The listing builds one solid part. Answer for the finished solid, in the listing's coordinates (mm). A direction names the side the tool comes from. Coordinates: 2 decimals unless noted, no trailing zeros. Order: outer loops, then holes, each group sorted by start corner. A loop starts at its lowest first (then second) coordinate and runs counter-clockwise, first axis right, second up. Notation, with made-up numbers: (27.25, 84) -> (79.25, 84) arc R18 ccw to (79.25, 98) -> close; hole circle Ø6 at (24.5, 25). An arc over 180 degrees is marked (long way). Answer in a Markdown table with one row per item. Add a question column.
```python
from build123d import *

# Parameters (mm, degrees)
BOSS_EXTRUDE1_DEPTH = 62
SKETCH5_W           = 26
SKETCH5_H           = 5
SKETCH5_W_2         = 5
SKETCH5_W_3         = 14.428632876
CUT_EXTRUDE1_DEPTH  = 106.090437243


with BuildPart() as part:
    # Sketch1 → Boss-Extrude1 (new body)
    with BuildSketch(Plane(origin=(0, 0, 0), x_dir=(1, 0, 0), z_dir=(0, 1, 0))):
        with BuildLine():
            Line((0, -7), (0, 7))
            ThreePointArc((0, 7), (1.464466094, 10.535533906), (5, 12))
            Line((5, 12), (68.215390309, 12))
            Line((68.215390309, 12), (81.5, 4.330127019))
            ThreePointArc((81.5, 4.330127019), (84, 0), (81.5, -4.330127019))
            Line((81.5, -4.330127019), (68.215390309, -12))
            Line((68.215390309, -12), (5, -12))
            ThreePointArc((5, -12), (1.464466094, -10.535533906), (0, -7))
        make_face()
    extrude(amount=BOSS_EXTRUDE1_DEPTH)

    # Sketch2 → Cut-Revolve1 (revolve, cut)
    with BuildSketch(Plane.XY):
        Polygon((48, 62), (48, 55.5), (49.5, 54), (48, 52.5), (48, 46), (37.5, 46), (36, 44.5), (34.5, 46), (24, 46), (24, 39.5), (25.5, 38), (24, 36.5), (24, 30), (13.5, 30), (12, 28.5), (10.5, 30), (0, 30), (-10, 30), (-10, 72), (48, 72), align=None)
    revolve(axis=Axis((89, 71.362230297, 0), (0, -1, 0)), mode=Mode.SUBTRACT)

    # Sketch5 → Cut-Revolve2 (revolve, cut)
    with BuildSketch(Plane.XY):
        with Locations((76, 2.5)):
            Rectangle(SKETCH5_W, SKETCH5_H)
        with Locations((57.5, 2.5)):
            Rectangle(SKETCH5_W_2, SKETCH5_H)
        with Locations((49.603587942, 2.5)):
            Rectangle(SKETCH5_W_2, SKETCH5_H)
        with Locations((41.707175883, 2.5)):
            Rectangle(SKETCH5_W_2, SKETCH5_H)
        with Locations((33.810763825, 2.5)):
            Rectangle(SKETCH5_W_2, SKETCH5_H)
        with Locations((25.914351767, 2.5)):
            Rectangle(SKETCH5_W_2, SKETCH5_H)
        with Locations((18.017939709, 2.5)):
            Rectangle(SKETCH5_W_2, SKETCH5_H)
        with Locations((5.303623271, 2.5)):
            Rectangle(SKETCH5_W_3, SKETCH5_H)
    revolve(axis=Axis((89, 64.780829091, 0), (0, -1, 0)), mode=Mode.SUBTRACT)

    # Sketch6 → Cut-Extrude1 (cut, through all)
    with BuildSketch(Plane(origin=(0, 0, 0), x_dir=(0, 0, -1), z_dir=(1, 0, 0))):
        with BuildLine():
            ThreePointArc((8.601411599, 11.928429193), (6.817380703, 12.222973886), (6, 13.835863095))
            Line((6, 13.835863095), (6, 20.164136905))
            ThreePointArc((6, 20.164136905), (6.817380703, 21.777026114), (8.601411599, 22.071570807))
            Line((8.601411599, 22.071570807), (12, 21))
            Line((12, 21), (12.955765894, 20.698648171))
            Line((12.955765894, 20.698648171), (12.955765894, 13.301351829))
            Line((12.955765894, 13.301351829), (12, 13))
            Line((12, 13), (8.601411599, 11.928429193))
        make_face()
        with BuildLine():
            Line((-6, 13.835863095), (-6, 20.164136905))
            ThreePointArc((-6, 20.164136905), (-6.817380703, 21.777026114), (-8.601411599, 22.071570807))
            Line((-8.601411599, 22.071570807), (-12, 21))
            Line((-12, 21), (-12.955765894, 20.698648171))
            Line((-12.955765894, 20.698648171), (-12.955765894, 13.301351829))
            Line((-12.955765894, 13.301351829), (-12, 13))
            Line((-12, 13), (-8.601411599, 11.928429193))
            ThreePointArc((-8.601411599, 11.928429193), (-6.817380703, 12.222973886), (-6, 13.835863095))
        make_face()
    extrude(amount=CUT_EXTRUDE1_DEPTH, mode=Mode.SUBTRACT)


solid = part.part
```
Q1. For faces 4 (the face through (63, 3, 0)), 5 (the face through (20.52, 2.54, 0.17)), 6 (the face through (48, 59, 0)), 7 (the face through (24.9, 37.4, 0.2)), 8 (the face through (36.666, 21.543, -10.277)), determine the directions among +Z, -Z, +X, -X, +Y, -Y from which every point of the face is accessible in a straight line to the end or side of a thin tool.
Q2. A cutting plane is placed at B-B (x = 72.5). Determine the outline of the cut face in (y, z), then the cut area to 3 significant figures.
Q3. Given pin 1 (4 mm diameter, centred on x = 11, z = -6.5, fed in from +Y); pin 2 (3 mm diameter, centred on x = 71.5, y = 51, fed in from -Z); pin 3 (7 mm diameter, centred on x = 51.5, y = 16, fed in from -Z); pin 4 (6 mm diameter, centred on x = 29.5, z = 6, fed in from +Y), each flat-ended and moving along its own axis, determine where each tip first touches the part or whether it passes through.
Q4. A cutting plane is placed at C-C (y = 35.5). Determine the outline of the cut face in (x, z), then the cut area to 3 significant figures.
Q5. Straight lines are drawn through the part: line 1 (Y direction, x = 42.5, z = -8); line 2 (Y direction, x = 25, z = 9.25) (3 decimals); line 3 (Z direction, x = 59, y = 19). For each, find the intervals that lie inside material, in ascending order.
Q6. A cutting plane is placed at A-A (y = 47.5). Determine the outline of the cut face in (x, z).
Q7. Determine the mould class of faces 1 (the face through (36.9, 45.4, 0.2)), 2 (the face through (22, 0, 0)), 3 (the face through (24, 43, 0)) for opening direction X: +X half, -X half, draft (parallel to the pull), parting line (faces both ways), or undercut.
Returned:
| question | item | result |
|---|---|---|
| 1 | face 4 | +X, -Y |
| 1 | face 5 | -Y |
| 1 | face 6 | -X, +Y |
| 1 | face 7 | -X |
| 1 | face 8 | +X, -X |
| 2 | outline | (5, -9.53) -> (12.22, -9.53) -> (11.93, -8.6) arc R2 cw to (13.84, -6) -> (20.16, -6) arc R2 cw to (22.07, -8.6) -> (21.78, -9.53) -> (62, -9.53) -> (62, 9.53) -> (21.78, 9.53) -> (22.07, 8.6) arc R2 cw to (20.16, 6) -> (13.84, 6) arc R2 cw to (11.93, 8.6) -> (12.22, 9.53) -> (5, 9.53) -> close |
| 2 | area | 1,020 mm² |
| 3 | pin 1 | stops at y = 30 |
| 3 | pin 2 | stops at z = -10.97 |
| 3 | pin 3 | stops at z = -12 |
| 3 | pin 4 | stops at y = 46 |
| 4 | outline | (25.12, -12) -> (68.22, -12) -> (81.5, -4.33) arc R5 ccw to (81.5, 4.33) -> (68.22, 12) -> (25.12, 12) arc R65 ccw to start |
| 4 | area | 1,280 mm² |
| 5 | line 1 | y = 5 to 11.84, 22.16 to 46 |
| 5 | line 2 | y = 5 to 12.133, 21.867 to 36.835, 39.165 to 46 |
| 5 | line 3 | z = -6 to 6 |
| 6 | outline | (49.8, -12) -> (68.22, -12) -> (81.5, -4.33) arc R5 ccw to (81.5, 4.33) -> (68.22, 12) -> (49.8, 12) arc R41 ccw to start |
| 7 | face 1 | undercut |
| 7 | face 2 | draft |
| 7 | face 3 | -X half |
